from build123d import *

# Parameters (mm, degrees)
SALIENTE_EXTRUIR1_DEPTH = 10
CROQUIS2_R              = 1.6
CORTAR_EXTRUIR1_DEPTH   = 10
CORTAR_EXTRUIR2_START   = 10
CROQUIS2_2_R            = 1.6
CORTAR_EXTRUIR2_DEPTH   = 10
CROQUIS3_R              = 3.75
CORTAR_EXTRUIR3_DEPTH   = 10


with BuildPart() as part:
    # Croquis1 → Saliente-Extruir1 (new body)
    with BuildSketch(Plane(origin=(0, 0, 0), x_dir=(0, 0, -1), z_dir=(1, 0, 0))):
        Polygon((-61.85, 0), (-66.85, 0), (-66.85, -3), (-54.85, -3), (-54.85, -6), (-54.85, -9), (54.85, -9), (54.85, -6), (54.85, -3), (66.85, -3), (66.85, 0), (61.85, 0), (51.85, 0), (51.85, -6), (-51.85, -6), (-51.85, 0), align=None)
    extrude(amount=SALIENTE_EXTRUIR1_DEPTH)

    # Croquis2 → Cortar-Extruir1 (cut)
    with BuildSketch(Plane(origin=(0, -6, 0), x_dir=(1, 0, 0), z_dir=(0, 1, 0))):
        with Locations((5, -61.85)):
            Circle(CROQUIS2_R)
        with Locations((5, 61.85)):
            Circle(CROQUIS2_R)
        with Locations(Location((5, -8.5, 0), (0, 0, 270))):
            Circle(CROQUIS2_R)
        with Locations(Location((5, 8.5, 0), (0, 0, 270))):
            Circle(CROQUIS2_R)
    extrude(amount=-CORTAR_EXTRUIR1_DEPTH, mode=Mode.SUBTRACT)

    # Croquis2_2 → Cortar-Extruir2 (cut)
    with BuildSketch(Plane(origin=(0, -6, 0), x_dir=(1, 0, 0), z_dir=(0, 1, 0)).offset(CORTAR_EXTRUIR2_START)):
        with Locations(Location((5, -61.85, 0), (0, 0, 90))):
            Circle(CROQUIS2_2_R)
        with Locations(Location((5, 61.85, 0), (0, 0, 90))):
            Circle(CROQUIS2_2_R)
        with Locations(Location((5, -8.5, 0), (0, 0, 270))):
            Circle(CROQUIS2_2_R)
        with Locations(Location((5, 8.5, 0), (0, 0, 270))):
            Circle(CROQUIS2_2_R)
    extrude(amount=-CORTAR_EXTRUIR2_DEPTH, mode=Mode.SUBTRACT)

    # Croquis3 → Cortar-Extruir3 (cut)
    with BuildSketch(Plane(origin=(0, -6, 0), x_dir=(1, 0, 0), z_dir=(0, 1, 0))):
        with Locations(Location((5, 0, 0), (0, 0, 270))):
            Circle(CROQUIS3_R)
    extrude(amount=-CORTAR_EXTRUIR3_DEPTH, mode=Mode.SUBTRACT)


solid = part.part
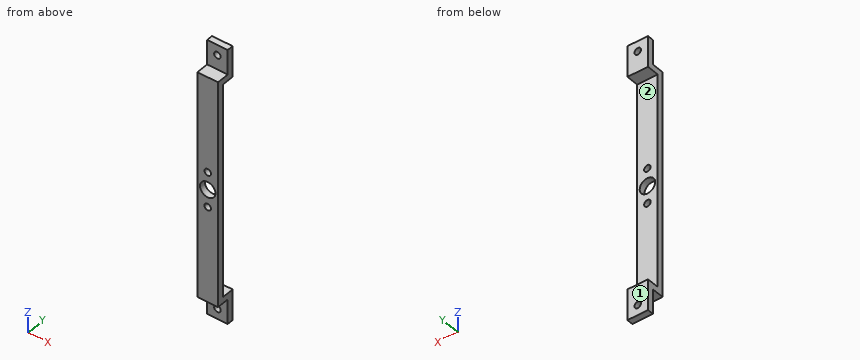
Read the model definition and answer for the solid it produces. Units are mm, in the model's axes. Face numbers are marked on the shaded views. Round coordinates to 2 decimals unless told otherwise and drop trailing zeros. Write each loop counter-clockwise with the first axis right and the second up, starting at its lowest first coordinate (ties: lowest second). Pieces come first, ordered by that corner, then holes.
Q1. Find section B-B on z = 61.85. Determine the outline of the cut face in (x, y), and give its area (3 significant figures).
Values:
outline: (0, -3) - (3.4, -3) - (3.4, 0) - (0, 0) - close; (6.6, -3) - (10, -3) - (10, 0) - (6.6, 0) - close
area: 20.4 mm2
Q2. Flat-ended cylindrical pins translate along their axes: P1, Ø3, axis at x = 7.5, z = -16.5, coming from the +Y side; P2, Ø3, axis at x = 3.5, z = 59, coming from the -Y side; P3, Ø4, axis at x = 1, z = -53.5, coming from the +Y side; P4, Ø3, axis at x = 3, y = -7, coming from the -Z side. Find the tip coordinate at first contact, or state that the pin passes through.
Values:
P1: stops at y = -6
P2: stops at y = -3
P3: stops at y = 0
P4: stops at z = -54.85
Q3. Find section D-D on z = -41. Determine the outline of the cut face in (x, y), and give its area (3 significant figures).
Values:
outline: (0, -9) - (10, -9) - (10, -6) - (0, -6) - close
area: 30.0 mm2
Q4. Find section A-A on x = 5. State how many separate pieces and enclosed holes the cut face has, and give its area (3 significant figures).
Values:
separate pieces: 6
enclosed holes: 0
area: 376 mm2
Q5. The mould has two halves that part along Z. Classify the marked faces 1 and 2: released by +Z, released by -Z, zero draft, split by the parting line, or undercut.
Values:
face 1: zero draft
face 2: undercut
Q6. Straight lines are drawn through the part: line 1 (Z direction, x = 5, y = -1.5); line 2 (X direction, y = -1.95, z = 61.85); line 3 (Z direction, x = 5.25, y = -5.5). For each, find the intervals that lie inside material, in ascending order.
Values:
line 1: z = -66.85 to -63.45, -60.25 to -51.85, 51.85 to 60.25, 63.45 to 66.85
line 2: x = 0 to 3.4, 6.6 to 10
line 3: z = -54.85 to -51.85, 51.85 to 54.85
Q7. Find section C-C on y = -4.5. Determine the outline of the cut face in (x, z), and give its area (3 significant figures).
Values:
outline: (0, -54.85) - (10, -54.85) - (10, -51.85) - (0, -51.85) - close; (0, 51.85) - (10, 51.85) - (10, 54.85) - (0, 54.85) - close
area: 60.0 mm2
